```python
from build123d import *

# Parameters (mm, degrees)
F0_W     = 130
F0_H     = 40
F1_DEPTH = 3
F2_W     = 3
F2_H     = 30
F3_DEPTH = 25
F5_DEPTH = 130.001


with BuildPart() as f1:
    # F0 (on Top) → F1 (new body)
    with BuildSketch(Plane.XY):
        with Locations((-2.750717, 31.965788)):
            Rectangle(F0_W, F0_H)
    extrude(amount=F1_DEPTH)

    # F2 (on face) → F3 (cut)
    with BuildSketch(Plane.XY.offset(3)):
        with Locations((-38.276677, 26.965788)):
            Rectangle(F2_W, F2_H)
        with Locations((-32.276677, 26.965788)):
            Rectangle(F2_W, F2_H)
        with Locations((-26.276677, 26.965788)):
            Rectangle(F2_W, F2_H)
        with Locations((-20.276677, 26.965788)):
            Rectangle(F2_W, F2_H)
        with Locations((-14.276677, 26.965788)):
            Rectangle(F2_W, F2_H)
        with Locations((-8.276677, 26.965788)):
            Rectangle(F2_W, F2_H)
        with Locations((-2.276677, 26.965788)):
            Rectangle(F2_W, F2_H)
        with Locations((3.723323, 26.965788)):
            Rectangle(F2_W, F2_H)
        with Locations((9.723323, 26.965788)):
            Rectangle(F2_W, F2_H)
        with Locations((15.723323, 26.965788)):
            Rectangle(F2_W, F2_H)
        with Locations((21.723323, 26.965788)):
            Rectangle(F2_W, F2_H)
        with Locations((27.723323, 26.965788)):
            Rectangle(F2_W, F2_H)
        with Locations((33.723323, 26.965788)):
            Rectangle(F2_W, F2_H)
        with Locations((39.723323, 26.965788)):
            Rectangle(F2_W, F2_H)
        with Locations((45.723323, 26.965788)):
            Rectangle(F2_W, F2_H)
        with Locations((51.723323, 26.965788)):
            Rectangle(F2_W, F2_H)
        with Locations((57.723323, 26.965788)):
            Rectangle(F2_W, F2_H)
    extrude(amount=-F3_DEPTH, mode=Mode.SUBTRACT)

    # F4 (on face) → F5 (cut, through all)
    with BuildSketch(Plane(origin=(-67.750717, 0, 0), x_dir=(0, -1, 0), z_dir=(-1, 0, 0))):
        Polygon((-18.210504, 3), (-11.965788, 2.4), (-11.965788, 3), align=None)
        Polygon((-11.965788, 0), (-11.965788, 0.6), (-18.210504, 0), align=None)
    extrude(amount=-F5_DEPTH, mode=Mode.SUBTRACT)


solid = f1.part
```
Design review of the part built by this model. Coordinates are the model's own, in mm. A direction names the side the tool comes from. Give positions to 0.01 mm unless a question says otherwise; leave off trailing zeros. Order: outer loops, then holes, each group sorted by start corner. A loop starts at its lowest first (then second) coordinate and runs counter-clockwise, first axis right, second up. Notation, with made-up numbers: (-33, -6) -> (-8, -6) arc R33 cw to (-8, 30) -> close; hole circle Ø9 at (58, 76.5). An arc over 180 degrees is marked (long way). Write each question's results on one line, items separated by ' | '. Start each with the question number.
Q1. Add section B-B on y = 20. State how many separate pieces and enclosed holes the cut face has, and give its area (3 significant figures).
Q2. Machinability: for faces 1 (the flat face through (-8, 41.966, 2)), 2 (the flat face through (30.702, 15.044, 0.304)), which of the approach directions +Z, -Z, +X, -X, +Y, -Y give a long, thin tool a straight path to every point of the face, cutting with its end or side? Answer none if there is none.
Q3. Wall thickness on L1, parallel to Y at x = 22.5, z = 0.85; L2, parallel to Z at x = 1.5, y = 16.5; L3, parallel to Z at x = -4, y = 14: over which ranges is each line inside the solid? List them lowest first. Write a range as from..to.
Q4. Add section A-A on x = -54. Give the boundary of the cut face in (y, z).
Q5. For pin 1 (0.9 mm diameter, centred on x = 4, z = 1, fed in from -Y), flat-tipped, find the tip position at first contact; note if it passes through.
Q6. Add section C-C on x = 9.5. Give the boundary of the cut face in (y, z), and give its area (3 significant figures).
Q7. Mouldability with a two-part tool opening along X and no side actions: class faces 3 (the flat face through (48.702, 15.044, 0.304)), 4 (the flat face through (-9.777, 27, 2)), 5 (the flat face through (-2, 41.966, 2)) as +X half, -X half, draft (parallel to the pull), parting line (faces both ways), or undercut.
Found:
1) separate pieces: 18 | enclosed holes: 0 | area: 237 mm2
2) face 1: +Z, -Z, -Y | face 2: -Z, +X, -X, -Y
3) L1: y = 41.97..51.97 | L2: z = 0.16..2.84 | L3: z = 0.4..2.6
4) outline: (11.97, 0.6) -> (18.21, 0) -> (51.97, 0) -> (51.97, 3) -> (18.21, 3) -> (11.97, 2.4) -> close
5) pin 1: stops at y = 41.97
6) outline: (41.97, 0) -> (51.97, 0) -> (51.97, 3) -> (41.97, 3) -> close | area: 30.0 mm2
7) face 3: draft | face 4: undercut | face 5: undercut
